Source: CAD feature listing. Evaluate the final solid. Frame: model axes, mm. A direction names the side the tool comes from. Coordinates: 2 decimals unless noted, no trailing zeros. Order: outer loops, then holes, each group sorted by start corner. A loop starts at its lowest first (then second) coordinate and runs counter-clockwise, first axis right, second up.
Item 1: Ray query, line 1 (Z direction, x = 0.5, y = 0); line 2 (Y direction, x = -18, z = -99); line 3 (Z direction, x = -7, y = 0.5). Return the intervals inside material, ascending.
Item 2: Section C-C on y = 5.5. Return the cut outline in (x, z) (3 decimals), then the cut area to 3 significant figures.
Item 3: Mould query, pull axis Z, two halves, no side actions, for faces 1 (the cylindrical face through (-15.21, -0.36, -91.15)), 2 (the cylindrical face through (0.112, 19.287, -27.938)), 3 (the cylindrical face through (0.7, 0.36, -120.64)), 4 (the cylindrical face through (11.165, -0.356, -76.602)). Classes: released by +Z, released by -Z, zero draft, split by the parting line, or undercut.
Item 4: Contact query for flat-ended pins moving along their axis: P1, Ø1, axis at x = 5, y = -6, coming from the +Z side; P2, Ø1, axis at x = 13, y = 0.5, coming from the +Z side; P3, Ø4.5, axis at x = 0, z = -25.4, coming from the +Y side; P4, Ø3, axis at y = -13, z = -90, coming from the +X side. Output: stop coordinate, or through.
Item 5: Section D-D on y = 0. Return the cut outline in (x, z) (3 decimals), then the cut area to 3 significant figures.
Item 6: Section B-B on z = -99.06. Return the cut outline in (x, y) (3 decimals), then the cut area to 3 significant figures.
Item 7: Reachability of faces 5 (the flat face through (9.525, 0, -41)), 6 (the flat face through (0, 25.4, -74)), 7 (the flat face through (-9.525, 0, -42)) from +Z, -Z, +X, -X, +Y, -Y: full face, straight path, thin tool, end or side. Return the list, or none.
Item 8: Section A-A on x = 4.5. Return the cut outline in (y, z), then the cut area to 3 significant figures.
from build123d import *

# Parameters (mm, degrees)
SKETCH1_R               = 17.145
SKETCH1_R_2             = 2.54
BOSS_EXTRUDE1_DEPTH     = 25.4
CUT_EXTRUDE1_DEPTH      = 128.160236415
CUT_EXTRUDE1_DEPTH_BACK = 128.160236415
SKETCH2_R               = 13.589
SKETCH2_R_2             = 2.54
FILLET1_R               = 25.4
FILLET2_R               = 25.4


with BuildPart() as part:
    # Sketch1 → Boss-Extrude1 (new, symmetric)
    with BuildSketch(Plane(origin=(0, 0, 0), x_dir=(1, 0, 0), z_dir=(0, 1, 0))):
        with BuildLine():
            Line((-9.525, 79.684694196), (-9.525, 0))
            Line((-9.525, 0), (9.525, 0))
            Line((9.525, 0), (9.525, 79.684694196))
            ThreePointArc((9.525, 79.684694196), (0, 120.65), (-9.525, 79.684694196))
        make_face()
        with Locations(Location((0, 99.06, 0), (0, 0, 270))):
            Circle(SKETCH1_R, mode=Mode.SUBTRACT)
        with Locations(Location((0, 25.4, 0), (0, 0, 270))):
            Circle(SKETCH1_R_2, mode=Mode.SUBTRACT)
    extrude(amount=BOSS_EXTRUDE1_DEPTH, both=True)

    # Sketch2 → Cut-Extrude1 (cut, two sides: drawn at the far end of the back side and taken through both)
    with BuildSketch(Plane(origin=(9.525, 0, 0), x_dir=(0, 0, -1), z_dir=(1, 0, 0)).offset(-CUT_EXTRUDE1_DEPTH_BACK)):
        with Locations((25.4, 0)):
            Circle(SKETCH2_R)
        with Locations((99.06, 0)):
            Circle(SKETCH2_R_2)
    extrude(amount=CUT_EXTRUDE1_DEPTH + CUT_EXTRUDE1_DEPTH_BACK, mode=Mode.SUBTRACT)

    # Fillet1
    # the kernel refuses this fillet: 25.4 mm, written as the material it takes off along each edge
    with BuildSketch(Plane(origin=(-73.025, -25.4, 0), x_dir=(0, 0, -1), z_dir=(1, 0, 0)), Plane(origin=(-73.025, 25.4, 0), x_dir=(0, -1, 0), z_dir=(1, 0, 0))) as fillet1_piece_1:
        with BuildLine():
            CenterArc((FILLET1_R, FILLET1_R), FILLET1_R, 180, 90)
            Line((0, FILLET1_R), (0, 0))
            Line((0, 0), (FILLET1_R, 0))
        make_face()
    extrude(amount=146.05, mode=Mode.SUBTRACT)

    # Fillet2
    fillet2_edges = [part.edges().sort_by_distance(p)[0] for p in [
        (9.525, 0, -79.684694196),
        (-9.525, 0, -79.684694196),
    ]]
    fillet(fillet2_edges, radius=FILLET2_R)


solid = part.part
Answer list:
1. line 1: z = -120.64 to -116.2, -81.92 to -38.99, -11.81 to 0
1. line 2: y = -25.4 to -2.54, 2.54 to 25.4
1. line 3: z = -119.48 to -114.71, -83.41 to -38.98, -11.82 to 0
2. outline: (-16.047, -84.616) arc R21.59 ccw (long way) to (16.047, -84.616) arc R25.4 cw to (9.525, -67.623) - (9.525, -37.826) - (-9.525, -37.826) - (-9.525, -67.623) arc R25.4 cw to start; (-9.525, -12.974) - (9.525, -12.974) - (9.525, -0.603) - (-9.525, -0.603) - close; hole circle Ø34.29 at (0, -99.06)
2. area: 1,580 mm2
3. face 1: undercut
3. face 2: undercut
3. face 3: split by the parting line
3. face 4: released by +Z
4. P1: stops at z = -0.6
4. P2: stops at z = -79.55
4. P3: passes through
4. P4: stops at x = 20.22
5. outline: (-21.44, -101.6) arc R21.59 ccw to (21.44, -101.6) - (16.956, -101.6) arc R17.145 cw to (-16.956, -101.6) - close; (-21.44, -96.52) - (-16.956, -96.52) arc R17.145 cw to (16.956, -96.52) - (21.44, -96.52) arc R21.59 ccw to (16.047, -84.616) arc R25.4 cw to (9.525, -67.623) - (9.525, -38.989) - (-9.525, -38.989) - (-9.525, -67.623) arc R25.4 cw to (-16.047, -84.616) arc R21.59 ccw to start; (-9.525, -11.811) - (9.525, -11.811) - (9.525, 0) - (-9.525, 0) - close
5. area: 1,500 mm2
6. outline: (-21.59, -25.4) - (-17.145, -25.4) - (-17.145, -2.54) - (-21.59, -2.54) - close; (-21.59, 2.54) - (-17.145, 2.54) - (-17.145, 25.4) - (-21.59, 25.4) - close; (17.145, -25.4) - (21.59, -25.4) - (21.59, -2.54) - (17.145, -2.54) - close; (17.145, 2.54) - (21.59, 2.54) - (21.59, 25.4) - (17.145, 25.4) - close
6. area: 406 mm2
7. face 5: +Z, +X, +Y, -Y
7. face 6: +Z, -Z, +X, -X, +Y
7. face 7: +Z, -X, +Y, -Y
8. outline: (-25.4, -120.18) - (25.4, -120.18) - (25.4, -115.6) - (-25.4, -115.6) - close; (-25.4, -82.52) - (25.4, -82.52) - (25.4, -25.4) arc R25.4 ccw to (-25.4, -25.4) - close; hole circle Ø27.18 at (0, -25.4)
8. area: 3,570 mm2
